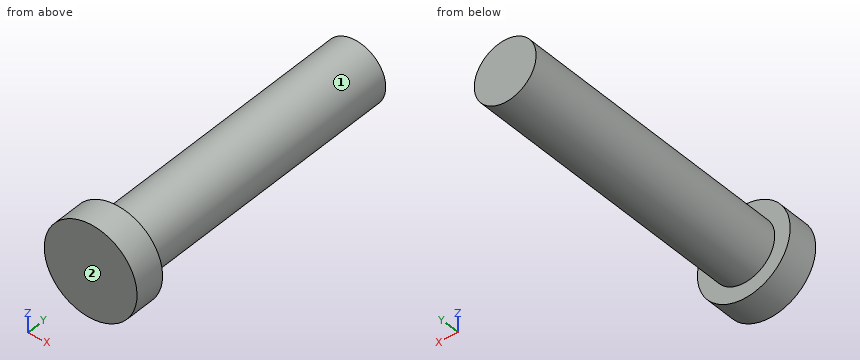
```python
from build123d import *

# Parameters (mm, degrees)
CROQUIS1_R              = 7.5
SALIENTE_EXTRUIR1_DEPTH = 5
CROQUIS2_R              = 5
SALIENTE_EXTRUIR2_DEPTH = 20
ESCALA1_SCALE           = 0.75
CROQUIS4_R              = 3.75
SALIENTE_EXTRUIR3_DEPTH = 20


with BuildPart() as part:
    # Croquis1 → Saliente-Extruir1 (new body)
    with BuildSketch(Plane(origin=(0, 0, 0), x_dir=(1, 0, 0), z_dir=(0, 1, 0))):
        with Locations(Location((0, 0, 0), (0, 0, 270))):
            Circle(CROQUIS1_R)
    extrude(amount=SALIENTE_EXTRUIR1_DEPTH)

    # Croquis2 → Saliente-Extruir2 (add)
    with BuildSketch(Plane(origin=(0, 5, 0), x_dir=(1, 0, 0), z_dir=(0, 1, 0))):
        with Locations(Location((0, 0, 0), (0, 0, 270))):
            Circle(CROQUIS2_R)
    extrude(amount=SALIENTE_EXTRUIR2_DEPTH)


with BuildPart() as part_1:
    # Escala1: scaled about (0, 10.5, 0)
    add(part.part.scale(ESCALA1_SCALE).moved(Location((0, 2.625, 0))))

    # Croquis4 → Saliente-Extruir3 (add)
    with BuildSketch(Plane(origin=(0, 21.375, 0), x_dir=(1, 0, 0), z_dir=(0, 1, 0))):
        with Locations(Location((0, 0, 0), (0, 0, 270))):
            Circle(CROQUIS4_R)
    extrude(amount=SALIENTE_EXTRUIR3_DEPTH)


solid = part_1.part
```
Could you check a few things on this model? Use its own coordinates, in mm. Face numbers are marked on the shaded views. A direction names the side the tool comes from. Round coordinates to 2 decimals unless told otherwise and drop trailing zeros. Write each loop counter-clockwise with the first axis right and the second up, starting at its lowest first coordinate (ties: lowest second). Pieces come first, ordered by that corner, then holes.
(1) Suppose I cut it at C-C on y = 29. Write out the boundary of the cut face in (x, z), and give its area (3 significant figures).
Findings below:
outline: circle Ø7.5 at (0, 0)
area: 44.2 mm2
(2) Which directions (+Z, -Z, +X, -X, +Y, -Y) give clear straight access to the entire face, cutting with the end or side of a thin tool? Please do the marked faces 1 and 2.
Findings below:
face 1: +Y
face 2: +Z, -Z, +X, -X, -Y
(3) For pin 1 (5 mm diameter, centred on x = -1.5, y = 11.5, fed in from +Z); pin 2 (2 mm diameter, centred on y = 34.5, z = 3.5, fed in from -X); pin 3 (2 mm diameter, centred on y = 17.5, z = -0.5, fed in from +X), each with a flat end and sliding along its axis, tell me the tip position at first contact or that it passes through.
Findings below:
pin 1: stops at z = 3.75
pin 2: stops at x = -2.8
pin 3: stops at x = 3.75
(4) Suppose I cut it at B-B on x = 0. Write out the boundary of the cut face in (y, z) (3 decimals), and give its area (3 significant figures).
Findings below:
outline: (2.625, -5.625) - (6.375, -5.625) - (6.375, -3.75) - (41.375, -3.75) - (41.375, 3.75) - (6.375, 3.75) - (6.375, 5.625) - (2.625, 5.625) - close
area: 305 mm2
(5) If I drill on probe 1 along Y at (x, z) = (2.5, 3.75) (3 decimals); probe 2 along X at (y, z) = (28, -1.25); probe 3 along X at (y, z) = (5, -3), over which ranges is the centre line in solid material (lowest first)?
Findings below:
probe 1: y = 2.625 to 6.375
probe 2: x = -3.54 to 3.54
probe 3: x = -4.76 to 4.76
(6) Suppose I cut it at A-A on z = 0. Write out the boundary of the cut face in (x, y) (3 decimals).
Findings below:
outline: (-5.625, 2.625) - (5.625, 2.625) - (5.625, 6.375) - (3.75, 6.375) - (3.75, 41.375) - (-3.75, 41.375) - (-3.75, 6.375) - (-5.625, 6.375) - close
(7) Suppose I cut it at D-D on x = -5. Write out the boundary of the cut face in (y, z) (3 decimals), and give its area (3 significant figures).
Findings below:
outline: (2.625, -2.577) - (6.375, -2.577) - (6.375, 2.577) - (2.625, 2.577) - close
area: 19.3 mm2
